The model under review builds one solid part; all positions refer to its coordinate system, in mm. A direction names the side the tool comes from. Coordinates: 2 decimals unless noted, no trailing zeros. Loops run counter-clockwise (first coordinate to the right, second up) from the corner with the lowest first, then second, coordinate; pieces in that order, holes last. Notation, with made-up numbers: (46.5, 73) - (62.5, 73) arc R31 cw to (62.5, 99) - close; hole circle Ø10 at (59.5, 51.5). An arc over 180 degrees is marked (long way). Answer in a Markdown table with one row per item. Add a question column.
(1) Mouldability with a two-part tool opening along X and no side actions: class faces 1 (the flat face through (36.108, 1, -9)), 2 (the flat face through (-0.4, 0, -6.6)), 3 (the flat face through (0, 1, -11.126)) as +X half, -X half, draft (parallel to the pull), parting line (faces both ways), or undercut.
(2) For line 1 along Z through (x, y) = (-19.5, 2); line 2 along X through (y, z) = (0.4, -6.5); line 3 along Z through (x, y) = (14.5, 0.2), list the stretches that pass through material, from the lowest coordinate up.
(3) We need section B-B on z = -2.5. Give the number of separate pieces and of enclosed holes in the cut face, plus the area to 3 significant figures.
(4) We need section D-D on x = -31. Write out the cut boundary in (y, z).
(5) Machinability: for faces 4 (the flat face through (-0.4, 3, -6.6)), 5 (the flat face through (-16, 1, -7.126)), which of the approach directions +Z, -Z, +X, -X, +Y, -Y give a long, thin tool a straight path to every point of the face, cutting with its end or side? Answer none if there is none.
(6) For P1, Ø1.5, axis at x = 13.5, z = -9, coming from the +Y side, flat-tipped, find the tip position at first contact; note if it passes through.
(7) We need section C-C on z = -10.5. Write out the cut boundary in (x, y), plus the area to 3 significant figures.
(8) We need section A-A on x = -12. Write out the cut boundary in (y, z).
from build123d import *

# Parameters (mm, degrees)
SKETCH1_R           = 2
SKETCH1_R_2         = 2.032942559
BOSS_EXTRUDE2_DEPTH = 3


with BuildPart() as part:
    # Sketch1 → Boss-Extrude2 (new body)
    # profile 1 of 4: a face of its own
    with BuildSketch(Plane(origin=(0, 0, 0), x_dir=(1, 0, 0), z_dir=(0, 1, 0))):
        with BuildLine():
            Line((-33.892215569, -2.874251497), (0.107784431, -2.874251497))
            Line((0.107784431, -2.874251497), (0.107784431, -0.874251497))
            ThreePointArc((0.107784431, -0.874251497), (-1.892215569, 1.125748503), (0.107784431, 3.125748503))
            Line((0.107784431, 3.125748503), (0.107784431, 7.125748503))
            Line((0.107784431, 7.125748503), (-4.428113954, 7.125748503))
            ThreePointArc((-4.428113954, 7.125748503), (-7.892215569, 5.125748503), (-11.356317184, 7.125748503))
            Line((-11.356317184, 7.125748503), (-20.428113954, 7.125748503))
            ThreePointArc((-20.428113954, 7.125748503), (-24.927491749, 5.262045198), (-27.892215569, 9.125748503))
            Line((-27.892215569, 9.125748503), (-29.892215569, 9.125748503))
            ThreePointArc((-29.892215569, 9.125748503), (-31.892215569, 7.125748503), (-33.892215569, 9.125748503))
            Line((-33.892215569, 9.125748503), (-35.892215569, 9.125748503))
            Line((-35.892215569, 9.125748503), (-35.892215569, -0.874251497))
            ThreePointArc((-35.892215569, -0.874251497), (-35.306429131, -2.288465059), (-33.892215569, -2.874251497))
        make_face()
        with Locations(Location((-31.892215569, 1.125748503, 0), (0, 0, 270))):
            Circle(SKETCH1_R, mode=Mode.SUBTRACT)
        with Locations(Location((-23.892215569, 1.125748503, 0), (0, 0, 270))):
            Circle(SKETCH1_R, mode=Mode.SUBTRACT)
        with Locations(Location((-15.892215569, 1.125748503, 0), (0, 0, 270))):
            Circle(SKETCH1_R_2, mode=Mode.SUBTRACT)
    # profile 2 of 4: a face of its own
    with BuildSketch(Plane(origin=(0, 0, 0), x_dir=(1, 0, 0), z_dir=(0, 1, 0))):
        with BuildLine():
            Line((0.107784431, 19.125748503), (0.107784431, 21.125748503))
            Line((0.107784431, 21.125748503), (-33.892215569, 21.125748503))
            ThreePointArc((-33.892215569, 21.125748503), (-35.306429131, 20.539962065), (-35.892215569, 19.125748503))
            Line((-35.892215569, 19.125748503), (-35.892215569, 9.125748503))
            Line((-35.892215569, 9.125748503), (-33.892215569, 9.125748503))
            ThreePointArc((-33.892215569, 9.125748503), (-31.892215569, 11.125748503), (-29.892215569, 9.125748503))
            Line((-29.892215569, 9.125748503), (-27.892215569, 9.125748503))
            ThreePointArc((-27.892215569, 9.125748503), (-24.927491749, 12.989451808), (-20.428113954, 11.125748503))
            Line((-20.428113954, 11.125748503), (-11.356317184, 11.125748503))
            ThreePointArc((-11.356317184, 11.125748503), (-7.892215569, 13.125748503), (-4.428113954, 11.125748503))
            Line((-4.428113954, 11.125748503), (0.107784431, 11.125748503))
            Line((0.107784431, 11.125748503), (0.107784431, 15.125748503))
            ThreePointArc((0.107784431, 15.125748503), (-1.892215569, 17.125748503), (0.107784431, 19.125748503))
        make_face()
        with Locations(Location((-31.892215569, 17.125748503, 0), (0, 0, 270))):
            Circle(SKETCH1_R, mode=Mode.SUBTRACT)
        with Locations(Location((-23.892215569, 17.125748503, 0), (0, 0, 270))):
            Circle(SKETCH1_R, mode=Mode.SUBTRACT)
        with Locations(Location((-15.892215569, 17.125748503, 0), (0, 0, 270))):
            Circle(SKETCH1_R_2, mode=Mode.SUBTRACT)
    # profile 3 of 4: a face of its own
    with BuildSketch(Plane(origin=(0, 0, 0), x_dir=(1, 0, 0), z_dir=(0, 1, 0))):
        with BuildLine():
            Line((36.107784431, 9.125748503), (34.107784431, 9.125748503))
            ThreePointArc((34.107784431, 9.125748503), (32.107784431, 7.125748503), (30.107784431, 9.125748503))
            Line((30.107784431, 9.125748503), (28.107784431, 9.125748503))
            ThreePointArc((28.107784431, 9.125748503), (25.143060612, 5.262045198), (20.643682816, 7.125748503))
            Line((20.643682816, 7.125748503), (11.571886046, 7.125748503))
            ThreePointArc((11.571886046, 7.125748503), (8.107784431, 5.125748503), (4.643682816, 7.125748503))
            Line((4.643682816, 7.125748503), (0.107784431, 7.125748503))
            Line((0.107784431, 7.125748503), (0.107784431, 3.125748503))
            ThreePointArc((0.107784431, 3.125748503), (1.521997994, 2.539962065), (2.107784431, 1.125748503))
            ThreePointArc((2.107784431, 1.125748503), (1.521997994, -0.288465059), (0.107784431, -0.874251497))
            Line((0.107784431, -0.874251497), (0.107784431, -2.874251497))
            Line((0.107784431, -2.874251497), (34.107784431, -2.874251497))
            ThreePointArc((34.107784431, -2.874251497), (35.521997994, -2.288465059), (36.107784431, -0.874251497))
            Line((36.107784431, -0.874251497), (36.107784431, 9.125748503))
        make_face()
        with Locations(Location((16.107784431, 1.125748503, 0), (0, 0, 270))):
            Circle(SKETCH1_R_2, mode=Mode.SUBTRACT)
        with Locations(Location((24.107784431, 1.125748503, 0), (0, 0, 270))):
            Circle(SKETCH1_R, mode=Mode.SUBTRACT)
        with Locations(Location((32.107784431, 1.125748503, 0), (0, 0, 270))):
            Circle(SKETCH1_R, mode=Mode.SUBTRACT)
    # profile 4 of 4: a face of its own
    with BuildSketch(Plane(origin=(0, 0, 0), x_dir=(1, 0, 0), z_dir=(0, 1, 0))):
        with BuildLine():
            ThreePointArc((30.107784431, 9.125748503), (32.107784431, 11.125748503), (34.107784431, 9.125748503))
            Line((34.107784431, 9.125748503), (36.107784431, 9.125748503))
            Line((36.107784431, 9.125748503), (36.107784431, 19.125748503))
            ThreePointArc((36.107784431, 19.125748503), (35.521997994, 20.539962065), (34.107784431, 21.125748503))
            Line((34.107784431, 21.125748503), (0.107784431, 21.125748503))
            Line((0.107784431, 21.125748503), (0.107784431, 19.125748503))
            ThreePointArc((0.107784431, 19.125748503), (1.521997994, 18.539962065), (2.107784431, 17.125748503))
            ThreePointArc((2.107784431, 17.125748503), (1.521997994, 15.711534941), (0.107784431, 15.125748503))
            Line((0.107784431, 15.125748503), (0.107784431, 11.125748503))
            Line((0.107784431, 11.125748503), (4.643682816, 11.125748503))
            ThreePointArc((4.643682816, 11.125748503), (8.107784431, 13.125748503), (11.571886046, 11.125748503))
            Line((11.571886046, 11.125748503), (20.643682816, 11.125748503))
            ThreePointArc((20.643682816, 11.125748503), (25.143060612, 12.989451808), (28.107784431, 9.125748503))
            Line((28.107784431, 9.125748503), (30.107784431, 9.125748503))
        make_face()
        with Locations(Location((16.107784431, 17.125748503, 0), (0, 0, 270))):
            Circle(SKETCH1_R_2, mode=Mode.SUBTRACT)
        with Locations(Location((24.107784431, 17.125748503, 0), (0, 0, 270))):
            Circle(SKETCH1_R, mode=Mode.SUBTRACT)
        with Locations(Location((32.107784431, 17.125748503, 0), (0, 0, 270))):
            Circle(SKETCH1_R, mode=Mode.SUBTRACT)
    extrude(amount=BOSS_EXTRUDE2_DEPTH)


solid = part.part
Outcome:
| question | item | result |
|---|---|---|
| 1 | face 1 | +X half |
| 1 | face 2 | draft |
| 1 | face 3 | undercut |
| 2 | line 1 | -21.13 to -11.13, -7.13 to 2.87 |
| 2 | line 2 | -35.89 to -26.91, -20.87 to -10.91, -4.87 to 5.09, 11.13 to 21.09, 27.13 to 36.11 |
| 2 | line 3 | -21.13 to -18.37, -15.88 to -11.13, -7.13 to -2.37, 0.12 to 2.87 |
| 3 | separate pieces | 8 |
| 3 | enclosed holes | 0 |
| 3 | area | 154 mm² |
| 4 | outline | (0, -21.13) - (3, -21.13) - (3, -18.92) - (0, -18.92) - close; (0, -15.34) - (3, -15.34) - (3, -10.92) - (0, -10.92) - close; (0, -7.34) - (3, -7.34) - (3, -2.92) - (0, -2.92) - close; (0, 0.66) - (3, 0.66) - (3, 2.87) - (0, 2.87) - close |
| 5 | face 4 | +Z, -Z, +X, -X, +Y |
| 5 | face 5 | +Y, -Y |
| 6 | P1 | through |
| 7 | outline | (-35.89, 0) - (-33.35, 0) - (-33.35, 3) - (-35.89, 3) - close; (-30.44, 0) - (-27.65, 0) - (-27.65, 3) - (-30.44, 3) - close; (27.86, 0) - (30.65, 0) - (30.65, 3) - (27.86, 3) - close; (33.56, 0) - (36.11, 0) - (36.11, 3) - (33.56, 3) - close |
| 7 | area | 32.0 mm² |
| 8 | outline | (0, -21.13) - (3, -21.13) - (3, -11.13) - (0, -11.13) - close; (0, -7.13) - (3, -7.13) - (3, 2.87) - (0, 2.87) - close |
